Answer from the drawing. Dimensions are ordinates in mm from the lowest x, y and z of the part. Give positions to 0.01 mm unless a question says otherwise; leave off trailing zeros. Write each loop counter-clockwise with the first axis right and the second up, starting at its lowest first coordinate (ties: lowest second). Pieces come first, ordered by that corner, then holes. Notation, with made-up numbers: M 83.5,-2.75 L 102.5,-2.75 A23 cw 102.5,14.25 Z; hole C 29.5,-13 d3. An arc over 180 degrees is marked long. Put each result on its own line as item: value.
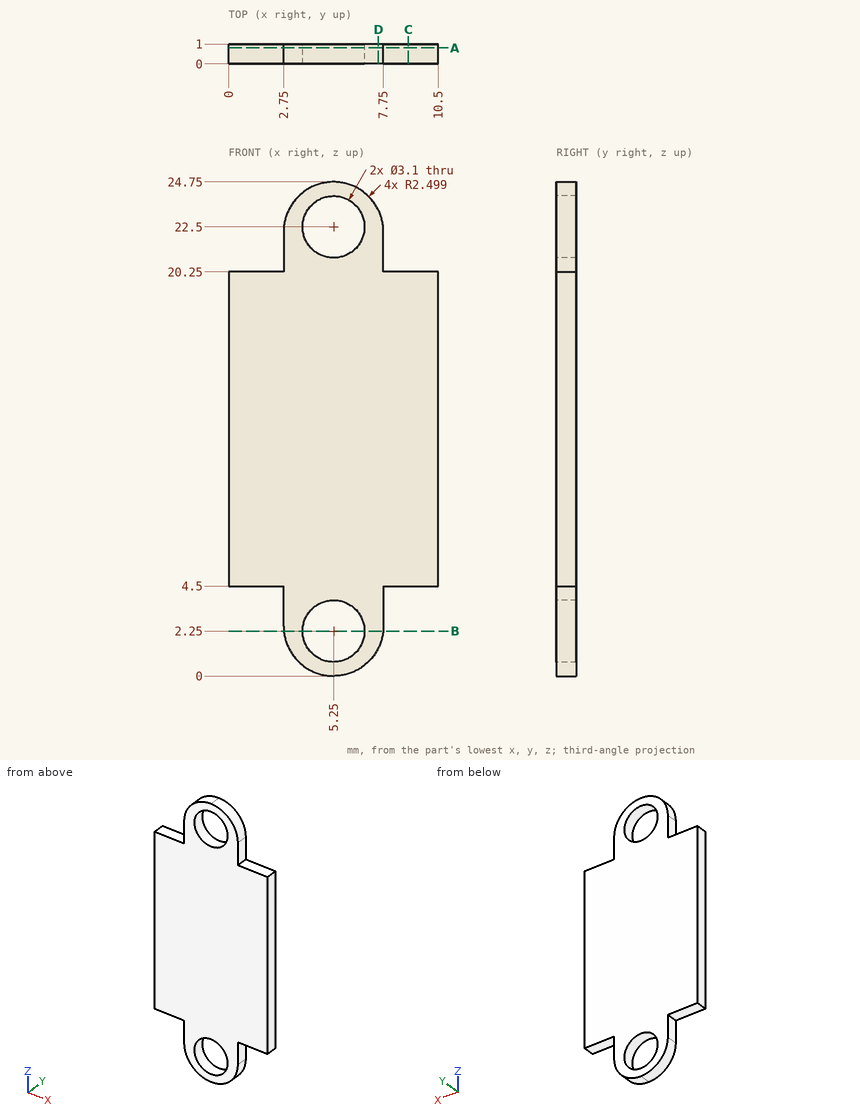
(1) Section D-D on x = 7.5 is taken. Determine the outline of the cut face in (y, z).
Result:
outline: M 0,1.41 L 1,1.41 L 1,23.34 L 0,23.34 Z
(2) Section A-A on y = 0.8 is taken. Give the number of separate pieces and of enclosed holes in the cut face, and give its area (3 significant figures).
Result:
separate pieces: 1
enclosed holes: 2
area: 190 mm²
(3) Section C-C on x = 9 is taken. Determine the outline of the cut face in (y, z).
Result:
outline: M 0,4.5 L 1,4.5 L 1,20.25 L 0,20.25 Z
(4) Straight lines are drawn through the part: line 1 along Z through (x, y) = (5.25, 0.6); line 2 along Z through (x, y) = (6.25, 0.35) (1 decimal); line 3 along Z through (x, y) = (10.25, 0.25). For each, find the intervals that lie inside material, in ascending order. Write a range as from..to.
Result:
line 1: z = 0..0.7, 3.8..20.95, 24.05..24.75
line 2: z = 0.2..1.1, 3.4..21.3, 23.7..24.5
line 3: z = 4.5..20.25
(5) Given pin 1 Ø1.5 at (x, z) = (4, 22) entering from +Y, flat-ended and moving along its own axis, determine where the tip first touches the part or whether it passes through.
Result:
pin 1: stops at y = 1
(6) Section B-B on z = 2.25 is taken. Determine the outline of the cut face in (x, y).
Result:
outline: M 2.76,0 L 3.7,0 L 3.7,1 L 2.76,1 Z; M 6.8,0 L 7.74,0 L 7.74,1 L 6.8,1 Z
